```python
from build123d import *

# Parameters (mm, degrees)
FASE1_SIZE                      = 1
FASE2_SIZE                      = 1
SKIZZE4_R                       = 2
AUFSATZ_LINEAR_AUSTRAGEN2_DEPTH = 2
VERRUNDUNG6_R                   = 2
AUFSATZ_LINEAR_START            = 2
SKIZZE5_R                       = 2
AUFSATZ_LINEAR_AUSTRAGEN3_DEPTH = 2
VERRUNDUNG7_R                   = 2
VERRUNDUNG8_R                   = 5


# Some blends are built 0.0001 mm under size
with BuildPart() as part:
    # Skizze2 → Rotation1 (revolve)
    with BuildSketch(Plane.XY, mode=Mode.PRIVATE) as rotation1_sk:
        with BuildLine():
            Line((-11.987410989, 29.669883346), (-11.987410989, 26.669883346))
            Line((-11.987410989, 26.669883346), (11.987410989, 26.669883346))
            Line((11.987410989, 26.669883346), (11.987410989, 29.669883346))
            ThreePointArc((11.987410989, 29.669883346), (0, 32), (-11.987410989, 29.669883346))
        make_face()
    revolve(rotation1_sk.sketch.rotate(Axis((-11.987410989, 26.669883346, 0), (1, 0, 0)), 180), axis=Axis((-11.987410989, 26.669883346, 0), (1, 0, 0)))

    # Fase1
    # the kernel refuses this chamfer: 5, 1 mm, written as the material it takes off along each edge
    with BuildSketch(Plane(origin=(-11.987410989, 26.669883346, 0), x_dir=(0, -1, 0), z_dir=(0, 0, 1))) as fase1_piece_1:
        with BuildLine():
            Line((4.195911394, 3.543317486), (3 - FASE1_SIZE, 0))
            Line((3 - FASE1_SIZE, 0), (3, 0))
            ThreePointArc((3, 0), (3.680793528, 1.846581965), (4.195911394, 3.543317486))
        make_face()
    revolve(axis=Axis((-11.987410989, 26.669883346, 0), (1, 0, 0)), mode=Mode.SUBTRACT)

    # Fase2
    # the kernel refuses this chamfer: 5, 1 mm, written as the material it takes off along each edge
    with BuildSketch(Plane(origin=(11.987410989, 26.669883346, 0), x_dir=(0, -1, 0), z_dir=(0, 0, 1))) as fase2_piece_1:
        with BuildLine():
            Line((4.195911394, -3.543317486), (3 - FASE2_SIZE, 0))
            Line((3 - FASE2_SIZE, 0), (3, 0))
            ThreePointArc((3, 0), (3.680793528, -1.846581965), (4.195911394, -3.543317486))
        make_face()
    revolve(axis=Axis((11.987410989, 26.669883346, 0), (1, 0, 0)), mode=Mode.SUBTRACT)

    # Skizze4 → Aufsatz-Linear austragen2 (add)
    with BuildSketch(Plane.ZY.offset(11.987410989)):
        with Locations(Location((0, 26.669883346, 0), (0, 0, 90))):
            Circle(SKIZZE4_R)
    extrude(amount=AUFSATZ_LINEAR_AUSTRAGEN2_DEPTH)

    # Verrundung6
    verrundung6_edges = [part.edges().sort_by_distance(p)[0] for p in [
        (-13.987410989, 24.669883346, 0),
    ]]
    fillet(verrundung6_edges, radius=VERRUNDUNG6_R - 0.0001)  # a hair under: the kernel refuses the full size

    # Skizze5 → Aufsatz-Linear austragen3 (add)
    with BuildSketch(Plane(origin=(11.987410989, 0, 0), x_dir=(0, 0, -1), z_dir=(1, 0, 0)).offset(AUFSATZ_LINEAR_START)):
        with Locations(Location((0, 26.669883346, 0), (0, 0, 270))):
            Circle(SKIZZE5_R)
    extrude(amount=-AUFSATZ_LINEAR_AUSTRAGEN3_DEPTH)

    # Verrundung7
    verrundung7_edges = [part.edges().sort_by_distance(p)[0] for p in [
        (13.987410989, 28.669883346, 0),
    ]]
    fillet(verrundung7_edges, radius=VERRUNDUNG7_R - 0.0001)  # a hair under: the kernel refuses the full size

    # Verrundung8
    verrundung8_edges = [part.edges().sort_by_distance(p)[0] for p in [
        (-8.444093503, 30.86579474, 0),
        (8.444093503, 30.86579474, 0),
    ]]
    fillet(verrundung8_edges, radius=VERRUNDUNG8_R)


solid = part.part
```
Source: CAD feature listing. Evaluate the final solid. Frame: model axes, mm. Round coordinates to 2 decimals unless told otherwise and drop trailing zeros. Loops run counter-clockwise (first coordinate to the right, second up) from the corner with the lowest first, then second, coordinate; pieces in that order, holes last.
1. Section query A-A on x = -11. Output: boundary loops of the cut face in (y, z), and give its area (3 significant figures).
2. Ray query, L1, parallel to Z at x = 8.25, y = 28.5; L2, parallel to Y at x = -8.25, z = 2.75; L3, parallel to Y at x = 7.5, z = 1. Return the intervals inside material, ascending.
3. Contact query for flat-ended pins moving along their axis: pin 1 (5 mm diameter, centred on x = -10, z = -3.5, fed in from -Y); pin 2 (2 mm diameter, centred on x = 9, z = -3, fed in from +Y); pin 3 (4 mm diameter, centred on y = 26, z = -4, fed in from -X). Output: stop coordinate, or through.
Answers below:
1. outline: circle Ø5.22 at (26.67, 0)
1. area: 21.4 mm2
2. L1: z = -3.8 to 3.8
2. L2: y = 23.48 to 29.86
2. L3: y = 22.35 to 30.99
3. pin 1: stops at y = 22.82
3. pin 2: stops at y = 30.19
3. pin 3: stops at x = -11.9
